Geometry: see drawing. Coordinates: mm, zero at the bounding-box minimum. Coordinates: 2 decimals unless noted, no trailing zeros. Loops run counter-clockwise (first coordinate to the right, second up) from the corner with the lowest first, then second, coordinate; pieces in that order, holes last. Notation, with made-up numbers: (71, 29.5) - (104, 29.5) arc R18 cw to (104, 34.5) - close; hole circle Ø2 at (-22, 47.5). An arc over 180 degrees is marked (long way). Answer in a Markdown table with one row per item.
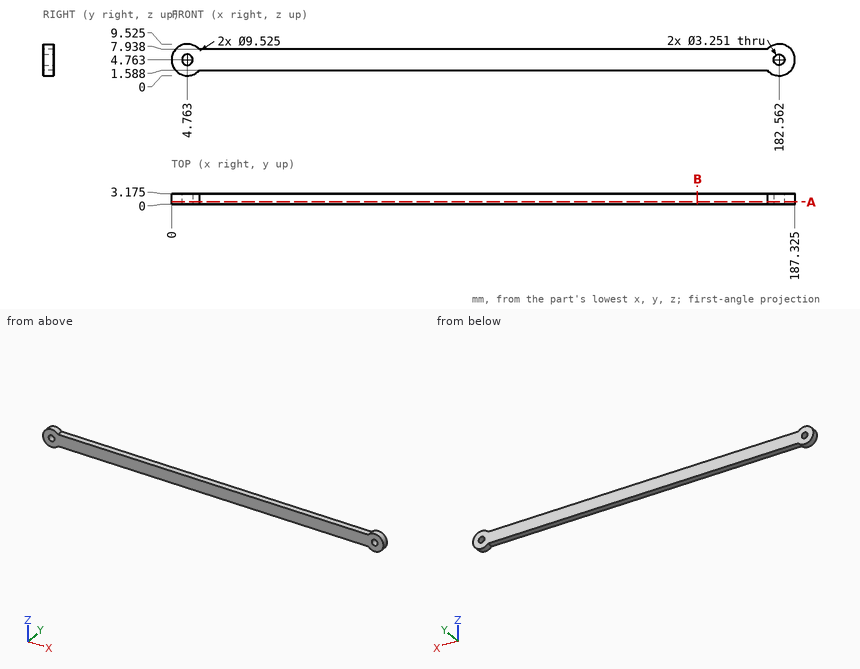
(1) Cut plane B-B on x = 158. Output: boundary loops of the cut face in (y, z) (1 decimal).
Verdict:
| item | result |
|---|---|
| outline | (0, 1.6) - (3.2, 1.6) - (3.2, 7.9) - (0, 7.9) - close |
(2) Cut plane A-A on y = 0.75. Output: boundary loops of the cut face in (x, z) (1 decimal).
Verdict:
| item | result |
|---|---|
| outline | (8.3, 1.6) - (179, 1.6) arc R4.8 ccw (long way) to (179, 7.9) - (8.3, 7.9) arc R4.8 ccw (long way) to start; hole circle Ø3.3 at (4.8, 4.8); hole circle Ø3.3 at (182.6, 4.8) |
(3) First-contact query: pin 1 Ø1 at (x, z) = (111, 2) entering from -Y; pin 2 Ø1 at (x, y) = (129, 2) entering from +Z; pin 3 Ø1 at (y, z) = (1, 6.5) entering from -X; pin 4 Ø1.6 at (x, y) = (74, 2) entering from -Z. Flat tips, straight axial feed; report the tip coordinate or a pass-through.
Verdict:
| item | result |
|---|---|
| pin 1 | stops at y = 0 |
| pin 2 | stops at z = 7.94 |
| pin 3 | stops at x = 0.16 |
| pin 4 | stops at z = 1.59 |
(4) Ray query, probe 1 along X at (y, z) = (0.55, 5.5) (1 decimal); probe 2 along Z at (x, y) = (122, 2.6); probe 3 along X at (y, z) = (1.5, 5.75) (1 decimal). Return the intervals inside material, ascending.
Verdict:
| item | result |
|---|---|
| probe 1 | x = 0.1 to 3.3, 6.2 to 181.1, 184 to 187.3 |
| probe 2 | z = 1.59 to 7.94 |
| probe 3 | x = 0.1 to 3.5, 6.1 to 181.3, 183.9 to 187.2 |
